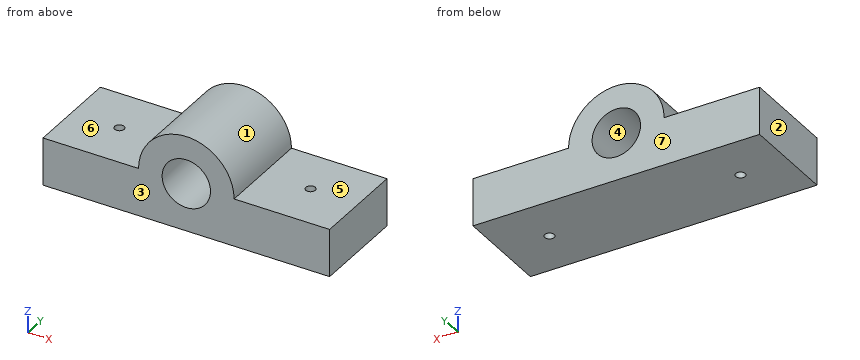
```python
from build123d import *

# Parameters (mm, degrees)
F1_DEPTH = 20
F2_R     = 1
F3_DEPTH = 25
F4_R     = 1
F5_DEPTH = 25


with BuildPart() as f1:
    # F0 (on Front) → F1 (new body)
    with BuildSketch(Plane.XZ):
        with BuildLine():
            Line((30, -5), (30, 5))
            Line((30, 5), (10, 5))
            ThreePointArc((10, 5), (7.0710678119, -2.0710678119), (0, -5))
            Line((0, -5), (30, -5))
        make_face()
        with BuildLine():
            ThreePointArc((0, -5), (-7.0710678119, -2.0710678119), (-10, 5))
            Line((-10, 5), (-30, 5))
            Line((-30, 5), (-30, -5))
            Line((-30, -5), (0, -5))
        make_face()
        with BuildLine():
            ThreePointArc((0, -5), (7.0710678119, -2.0710678119), (10, 5))
            Line((10, 5), (5.0676797819, 5))
            ThreePointArc((5.0676797819, 5), (0, -0.0676797819), (-5.0676797819, 5))
            Line((-5.0676797819, 5), (-10, 5))
            ThreePointArc((-10, 5), (-7.0710678119, -2.0710678119), (0, -5))
        make_face()
        with BuildLine():
            Line((5.0676797819, 5), (10, 5))
            ThreePointArc((10, 5), (0, 15), (-10, 5))
            Line((-10, 5), (-5.0676797819, 5))
            ThreePointArc((-5.0676797819, 5), (0, 10.0676797819), (5.0676797819, 5))
        make_face()
    extrude(amount=F1_DEPTH)

    # F2 (on face) → F3 (cut)
    with BuildSketch(Plane.XY.offset(5)):
        with Locations((-20, -10)):
            Circle(F2_R)
    extrude(amount=-F3_DEPTH, mode=Mode.SUBTRACT)

    # F4 (on face) → F5 (cut)
    with BuildSketch(Plane.XY.offset(5)):
        with Locations((20, -10)):
            Circle(F4_R)
    extrude(amount=-F5_DEPTH, mode=Mode.SUBTRACT)


solid = f1.part
```
Geometry: final body of the model. Coordinates: model frame, mm. Face numbers are marked on the shaded views. A direction names the side the tool comes from. Coordinates: 2 decimals unless noted, no trailing zeros. Order: outer loops, then holes, each group sorted by start corner. A loop starts at its lowest first (then second) coordinate and runs counter-clockwise, first axis right, second up. Notation, with made-up numbers: (38.5, 56.25) -> (60.5, 56.25) arc R18 cw to (60.5, 64.25) -> close; hole circle Ø6 at (-7.75, 38.25). An arc over 180 degrees is marked (long way). Answer in a Markdown table with one row per item.
Item 1: Section A-A on x = 20. Output: boundary loops of the cut face in (y, z).
Return value:
| item | result |
|---|---|
| outline | (-20, -5) -> (-11, -5) -> (-11, 5) -> (-20, 5) -> close; (-9, -5) -> (0, -5) -> (0, 5) -> (-9, 5) -> close |
Item 2: Draft query along X for the marked faces 1, 2, 3 and 4. Return one class per face: released by +X, released by -X, zero draft, split by the parting line, or undercut.
Return value:
| item | result |
|---|---|
| face 1 | split by the parting line |
| face 2 | released by -X |
| face 3 | zero draft |
| face 4 | undercut |
Item 3: Section D-D on x = 0. Output: boundary loops of the cut face in (y, z), plus the area to 3 significant figures.
Return value:
| item | result |
|---|---|
| outline | (-20, -5) -> (0, -5) -> (0, -0.07) -> (-20, -0.07) -> close; (-20, 10.07) -> (0, 10.07) -> (0, 15) -> (-20, 15) -> close |
| area | 197 mm² |
Item 4: Section B-B on z = 4.25. Output: boundary loops of the cut face in (x, y).
Return value:
| item | result |
|---|---|
| outline | (-30, -20) -> (-5.01, -20) -> (-5.01, 0) -> (-30, 0) -> close; (5.01, -20) -> (30, -20) -> (30, 0) -> (5.01, 0) -> close; hole circle Ø2 at (-20, -10); hole circle Ø2 at (20, -10) |
Item 5: Access query for the marked faces 5, 6 and 7. Directions: +Z, -Z, +X, -X, +Y, -Y. A direction counts if a zero-diameter tool reaches every point of the face in a straight line with its end or side. Return the directions, or none.
Return value:
| item | result |
|---|---|
| face 5 | +Z, +X, +Y, -Y |
| face 6 | +Z, -X, +Y, -Y |
| face 7 | +Z, -Z, +X, -X, +Y |
Item 6: Section C-C on y = -8. Output: boundary loops of the cut face in (x, z), plus the area to 3 significant figures.
Return value:
| item | result |
|---|---|
| outline | (-30, -5) -> (30, -5) -> (30, 5) -> (10, 5) arc R10 ccw to (-10, 5) -> (-30, 5) -> close; hole circle Ø10.14 at (0, 5) |
| area | 676 mm² |
Item 7: Contact query for flat-ended pins moving along their axis: P1, Ø4, axis at y = -6, z = 12, coming from the -X side; P2, Ø8, axis at x = 0, z = 5, coming from the -Y side; P3, Ø6, axis at x = -4.5, y = -6.5, coming from the +Z side; P4, Ø5, axis at y = -2, z = 9, coming from the -X side. Output: stop coordinate, or through.
Return value:
| item | result |
|---|---|
| P1 | stops at x = -8.66 |
| P2 | passes through |
| P3 | stops at z = 14.89 |
| P4 | stops at x = -9.89 |
Item 8: Ray query, L1, parallel to Y at x = 20, z = 1; L2, parallel to Z at x = -23, y = -4; L3, parallel to X at y = -5.5, z = 7. Return the intervals inside material, ascending.
Return value:
| item | result |
|---|---|
| L1 | y = -20 to -11, -9 to 0 |
| L2 | z = -5 to 5 |
| L3 | x = -9.8 to -4.66, 4.66 to 9.8 |
